Autodesk Inventor part; units mm, degrees
ref_plane "YZ Plane" through (0, 0, 0) normal (1, 0, 0) x (0, 1, 0)
ref_plane "XZ Plane" through (0, 0, 0) normal (0, 1, 0) x (-1, 0, 0)
ref_plane "XY Plane" through (0, 0, 0) normal (0, 0, 1) x (1, 0, 0)
sketch "Esboço1" plane through (0, 0, 0) normal (0, 0, 1) x (1, 0, 0)
  circle A0 centre (0, 0) radius 24
  dimension "d0" = 48
extrude "Extrusão1" add sketch "Esboço1" along normal blind 6
sketch "Esboço2" plane through (0, 0, 6) normal (0, 0, 1) x (1, 0, 0)
  circle A0 centre (0, 0) radius 24
  circle A1 centre (0, 0) radius 10
  dimension "d3" = 20
extrude "Extrusão2" add sketch "Esboço2" along normal blind 10 contours A1
sketch "Esboço3" plane through (0, 0, 0) normal (0, 0, -1) x (-1, 0, 0)
  circle A0 centre (0, 0) radius 24
  circle A1 centre (0, 0) radius 14
  dimension "d6" = 28
extrude "Extrusão3" add sketch "Esboço3" along normal blind 4 contours A1
sketch "Esboço4" plane through (0, 0, -4) normal (0, 0, -1) x (-1, 0, 0)
  circle A0 centre (0, 0) radius 14
  circle A1 centre (0, 0) radius 10
  dimension "d9" = 20
extrude "Extrusão4" add sketch "Esboço4" along normal blind 20 contours A1
sketch "Esboço5" plane through (0, 0, 0) normal (1, 0, 0) x (0, 1, 0)
  line L0 (10, -20) -> (9.5, -20)
  line L1 (9.5, -20) -> (9.5, -21.25)
  line L2 (9.5, -21.25) -> (10, -21.25)
  line L3 (10, -21.25) -> (10, -20)
  line L4 (-10, -24) -> (10, -24)
  line L5 (0, -32) -> (0, 24)
  point P0 (0, 0)
  dimension "d12" = 1.25
  dimension "d13" = 4
  dimension "d14" = 9.5
revolve "Revolução1" cut sketch "Esboço5" angle 360 about axis through (0, 0, -10) along (0, 0, 1)
sketch "Esboço6" plane through (0, 0, 0) normal (0, 0, -1) x (-1, 0, 0)
  circle A0 centre (0, 0) radius 14
  point P0 (19, 0)
  dimension "d16" = 19
hole "Furo1" at (-19, 0, 0) direction (0, 0, 1) diameter 4.5 end through all counterbore diameter 8 counterbore depth 4.5
pattern_circular "Padrão circular1" count 4 over 360 about axis through (0, 0, 0) along (0, 0, 1) of "Furo1"
chamfer "Chanfro1" distance 0.5 angle 45 5 edges at (-10, 0, 16) (-24, 0, 6) (-24, 0, 0) (14, 0, -4) (10, 0, -24)
Verification items for the finished model (mm, model axes). A direction names the side the tool comes from. Give positions to 0.01 mm unless a question says otherwise; leave off trailing zeros. Write each loop counter-clockwise with the first axis right and the second up, starting at its lowest first coordinate (ties: lowest second). Pieces come first, ordered by that corner, then holes. Notation, with made-up numbers: M 86,50 L 91,50 A9 cw 91,58 Z; hole C 10,80.5 d1. An arc over 180 degrees is marked long. Put each result on its own line as item: value. Start each with the question number.
1. Section check D-D (z = -8). Record the cut outline in (x, y).
2. Draft check along Y on faces 4 (the face through (-12.932, 5.362, -1.726)), 5 (the face through (9, -5, -4)), 6 (the face through (-22.966, -0.521, 2.282)). Enter one of: +Y half, -Y half, draft (parallel to the pull), parting line (faces both ways), or undercut.
3. Scan lines: line 1 along Y through (x, z) = (0, 5.2); line 2 along X through (y, z) = (-2.5, 4); line 3 along Z through (x, y) = (-18.5, 14.5). Record each from-to range of solid material in increasing order. Write a range as [from, to].
4. Section check A-A (z = 1.5). Record the cut outline in (x, y).
5. Set-up check for faces 1 (the face through (10.1, -10.1, 0)), 2 (the face through (10, -5, 6)), 3 (the face through (-8.43, 4.38, -20.63)): record each of +Z, -Z, +X, -X, +Y, -Y from which the full face is reachable in a straight line by a thin tool's end or side.
6. Go/stop test with flat-tipped pins: pin 1 Ø9 at (x, y) = (-19, 0.5) entering from -Z; pin 2 Ø2 at (y, z) = (9, 11.5) entering from -X; pin 3 Ø10 at (y, z) = (15, 0) entering from +X; pin 4 Ø4 at (x, y) = (19, 0) entering from -Z. Record where each tip stops, or that it passes through.
7. Section check B-B (y = 0). Give the number of separate pieces and of enclosed holes in the cut face, and give its area (3 significant figures).
Answer list:
1. outline: C 0,0 d20
2. face 4: parting line
2. face 5: draft
2. face 6: undercut
3. line 1: [-24, -21.25], [-16.75, 16.75], [21.25, 24]
3. line 2: [-23.87, -22.12], [-15.88, 15.88], [22.12, 23.87]
3. line 3: [0.01, 5.99]
4. outline: C 0,0 d48; hole C -19,0 d8; hole C 0,-19 d8; hole C 0,19 d8; hole C 19,0 d8
5. face 1: -Z
5. face 2: +Z
5. face 3: none
6. pin 1: z = 0
6. pin 2: x = -6
6. pin 3: x = 21.81
6. pin 4: through
7. separate pieces: 3
7. enclosed holes: 0
7. area: 912 mm2
